For this review, take the finished solid that the model builds, in its own axes (mm). Face numbers are marked on the shaded views. A direction names the side the tool comes from. Round coordinates to 2 decimals unless told otherwise and drop trailing zeros. Write each loop counter-clockwise with the first axis right and the second up, starting at its lowest first coordinate (ties: lowest second). Pieces come first, ordered by that corner, then holes. Notation, with made-up numbers: M 51,28.5 L 60,28.5 A21 ccw 60,65.5 Z; hole C 73.5,5 d10. An arc over 180 degrees is marked long. Write each question's results on one line, items separated by ' | '. Start each with the question number.
```python
from build123d import *

# Parameters (mm, degrees)
F0_R           = 1.016
F0_W           = 20.32
F0_H           = 40.64
F2_DEPTH       = 17.526
F3_START       = -25.4
F3_DEPTH       = 40.641
F4_R           = 3.81
F5_DEPTH       = 6.35
F7_D           = 2.032
F7_CSINK_D     = 3.175
F7_CSINK_ANGLE = 82


with BuildPart() as f2:
    # F0 (on Top) → F2 (new body, through all)
    with BuildSketch(Plane.XY):
        with BuildLine():
            Line((-15.24, 13.97), (-15.24, -40.64))
            Line((-15.24, -40.64), (15.24, -40.64))
            Line((15.24, -40.64), (15.24, 13.97))
            Line((15.24, 13.97), (7.5805170802, 27.2366135768))
            ThreePointArc((7.5805170802, 27.2366135768), (0, 31.6132271537), (-7.5805170802, 27.2366135768))
            Line((-7.5805170802, 27.2366135768), (-15.24, 13.97))
        make_face()
        with Locations((-5.4991, -34.036)):
            Circle(F0_R, mode=Mode.SUBTRACT)
        with Locations((5.4991, -34.036)):
            Circle(F0_R, mode=Mode.SUBTRACT)
        with Locations((0, -10.16)):
            Rectangle(F0_W, F0_H, mode=Mode.SUBTRACT)
        with Locations((-5.4991, 13.97)):
            Circle(F0_R, mode=Mode.SUBTRACT)
        with Locations((5.4991, 13.97)):
            Circle(F0_R, mode=Mode.SUBTRACT)
    extrude(amount=-F2_DEPTH)

    # F1 (on Right) → F3 (intersect)
    with BuildSketch(Plane.YZ.offset(F3_START)):
        Polygon((21.3039489306, 0), (-40.64, 0), (-40.64, -6.35), (10.053559014, -6.35), (16.4474982036, -13.97), (16.4474982036, -17.526), (31.6132271537, -17.526), (31.6132271537, -12.2861193594), align=None)
    extrude(amount=F3_DEPTH, mode=Mode.INTERSECT)

    # F4 (on face) → F5 (join)
    with BuildSketch(Plane(origin=(0, 0, -17.526), x_dir=(1, 0, 0), z_dir=(0, 0, -1))):
        with Locations((0, -22.86)):
            Circle(F4_R)
    extrude(amount=F5_DEPTH)

    # F7 (through all)
    with Locations(Plane(origin=(0, 0, -23.876), x_dir=(1, 0, 0), z_dir=(0, 0, -1))):
        with Locations((0, -22.86)):
            CounterSinkHole(F7_D / 2, F7_CSINK_D / 2, counter_sink_angle=F7_CSINK_ANGLE)


solid = f2.part
```
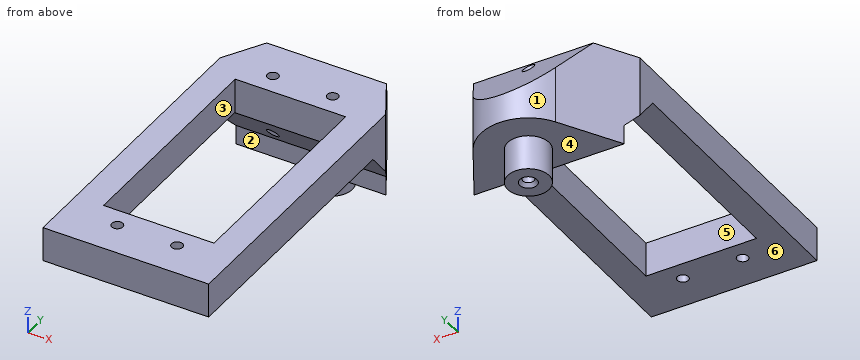
Item 1: We need section B-B on x = 0. State the section outline as (y, z) points, then the cut area to 3 significant figures.
Item 2: Mouldability with a two-part tool opening along Y and no side actions: class the marked faces 1, 2 and 3 as pulls with the +Y half, pulls with the -Y half, needs draft (parallel to the pull), parting line crosses it, or undercut.
Item 3: Insertion check: P1, Ø7, axis at x = -0.5, z = -4, coming from the +Y side; P2, Ø2.5, axis at x = -5.5, y = -34.04, coming from the -Z side; P3, Ø1.5, axis at x = -1, z = -19, coming from the -Y side. Each pin has a flat end and moves straight along its axis. Give the tip position at first contact, or say it passes through.
Item 4: We need section A-A on y = -15. State the section outline as (x, z) points.
Item 5: We need section D-D on z = -20.25. State the section outline as (x, y) points, then the cut area to 3 significant figures.
Item 6: For the marked faces 4, 5 and 6, list the 3-axis set-ups (+Z, -Z, +X, -X, +Y, -Y) from which the entire face can be reached by the end or side of a thin tool; tool diameter is ignored.
Item 7: For probe 1 along X at (y, z) = (13.97, -8.25); probe 2 along Y at (x, z) = (0.5, -3.75); probe 3 along Y at (x, z) = (-5, -4.25), list the stretches that pass through material, from the lowest coordinate up.
Item 8: We need section C-C on z = -9.5. State the section outline as (x, y) points.
Numbers:
1) outline: M -40.64,-6.35 L -30.48,-6.35 L -30.48,0 L -40.64,0 Z; M 10.16,-6.48 L 16.45,-13.97 L 16.45,-17.53 L 19.05,-17.53 L 19.05,-23.88 L 21.27,-23.88 L 21.84,-23.22 L 21.84,-0.64 L 21.3,0 L 10.16,0 Z; M 23.88,-23.22 L 24.45,-23.88 L 26.67,-23.88 L 26.67,-17.53 L 31.61,-17.53 L 31.61,-12.29 L 23.88,-3.07 Z | area: 335 mm^2
2) face 1: pulls with the +Y half | face 2: pulls with the -Y half | face 3: undercut
3) P1: stops at y = 27.6 | P2: stops at z = -6.35 | P3: stops at y = 19.06
4) outline: M -15.24,-6.35 L -10.16,-6.35 L -10.16,0 L -15.24,0 Z; M 10.16,-6.35 L 15.24,-6.35 L 15.24,0 L 10.16,0 Z
5) outline: C 0,22.86 d7.62; hole C 0,22.86 d2.03 | area: 42.4 mm^2
6) face 4: -Z | face 5: +Z, -Z | face 6: -Z, +X, -X, -Y
7) probe 1: x = -15.24 to -6.52, -4.48 to 4.48, 6.52 to 15.24 | probe 2: y = -40.64 to -30.48, 10.16 to 21.98, 23.74 to 24.45 | probe 3: y = -40.64 to -34.92, -33.15 to -30.48, 10.16 to 13.09, 14.85 to 24.87
8) outline: M -15.24,12.7 L 15.24,12.7 L 15.24,13.97 L 7.58,27.24 A8.75 ccw 5.95,29.28 L -5.95,29.28 A8.75 ccw -7.58,27.24 L -15.24,13.97 Z; hole C -5.5,13.97 d2.03; hole C 0,22.86 d2.03; hole C 5.5,13.97 d2.03
